Can you work these out from the model? Positions are in its coordinate system, mm. Face numbers are marked on the shaded views. A direction names the side the tool comes from. Give positions to 0.01 mm unless a question says otherwise; leave off trailing zeros. Write each loop counter-clockwise with the first axis right and the second up, starting at its lowest first coordinate (ties: lowest second). Pieces come first, ordered by that corner, then holes.
1. Suppose I cut it at D-D (y = -23.5). Please give me the cut outline in (x, z) (3 decimals).
2. Suppose I cut it at B-B (y = 0). Please give me the cut outline in (x, z) (3 decimals), and give its area (3 significant figures).
3. I'm going to push flat-ended pins straight in: pin 1 (11.5 mm diameter, centred on y = -14.5, z = -29, fed in from -X); pin 2 (18 mm diameter, centred on x = 13.5, y = -4, fed in from -Z) (3 decimals); pin 3 (20 mm diameter, centred on x = -42, y = -6.5, fed in from +Z); pin 4 (12 mm diameter, centred on x = -44, z = -33.5, fed in from -Y). Where does each tip first touch, or does it pass through?
4. Suppose I cut it at A-A (x = -23.5). Please give me the cut outline in (y, z) (3 decimals).
5. Suppose I cut it at C-C (x = 0). Please give me the cut outline in (y, z) (3 decimals).
6. On a 3-axis mill with a long thin cutter (end or side, diameter ignored), from which of +Z, -Z, +X, -X, +Y, -Y can I reach the whole of each face in a straight line? I mean the marked faces 1, 2 and 3. Say none if no direction works.
7. If I drill on probe 1 along Y at (x, z) = (-23.5, -1.95); probe 2 along X at (y, z) = (23.5, -1.85); probe 3 along X at (y, z) = (23.5, -1.6), over which ranges is the centre line in solid material (lowest first)?
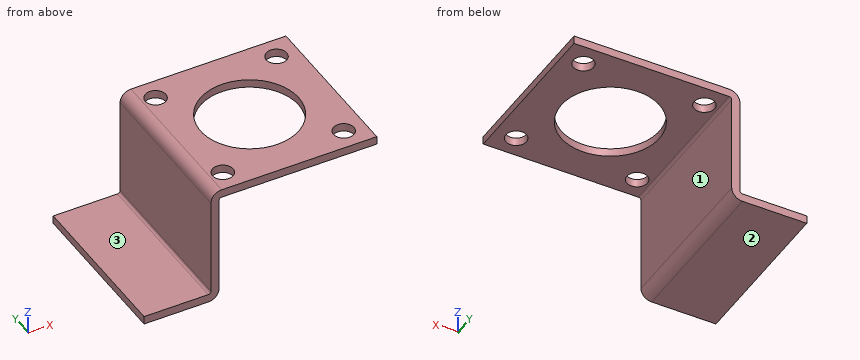
```python
from build123d import *

# Parameters (mm, degrees)
BOSS_EXTRUDE1_DEPTH     = 31.75
CUT_EXTRUDE1_DEPTH      = 82.262795763
CUT_EXTRUDE1_DEPTH_BACK = 82.262795763
SKETCH1_R               = 19.05
SKETCH1_R_2             = 4


with BuildPart() as part:
    # Sketch2 → Boss-Extrude1 (new, symmetric)
    with BuildSketch(Plane(origin=(0, 0, 0), x_dir=(1, 0, 0), z_dir=(0, 1, 0))):
        with BuildLine():
            Line((31.75, 0), (-28.499943, 0))
            ThreePointArc((-28.499943, 0), (-31.46342752, 1.22751548), (-32.690943, 4.191))
            Line((-32.690943, 4.191), (-32.690943, 42.208958))
            ThreePointArc((-32.690943, 42.208958), (-32.98852251, 42.92737849), (-33.706943, 43.224958))
            Line((-33.706943, 43.224958), (-58.673873, 43.224958))
            Line((-58.673873, 43.224958), (-58.673873, 46.399958))
            Line((-58.673873, 46.399958), (-33.706943, 46.399958))
            ThreePointArc((-33.706943, 46.399958), (-30.74345848, 45.17244252), (-29.515943, 42.208958))
            Line((-29.515943, 42.208958), (-29.515943, 4.191))
            ThreePointArc((-29.515943, 4.191), (-29.21836349, 3.47257951), (-28.499943, 3.175))
            Line((-28.499943, 3.175), (31.75, 3.175))
            Line((31.75, 3.175), (31.75, 0))
        make_face()
    extrude(amount=BOSS_EXTRUDE1_DEPTH, both=True)

    # Sketch1 → Cut-Extrude1 (cut, two sides: drawn at the far end of the back side and taken through both)
    with BuildSketch(Plane.XY.offset(-CUT_EXTRUDE1_DEPTH_BACK)):
        Circle(SKETCH1_R)
        with Locations((23.5, 23.5)):
            Circle(SKETCH1_R_2)
        with Locations((23.5, -23.5)):
            Circle(SKETCH1_R_2)
        with Locations((-23.5, -23.5)):
            Circle(SKETCH1_R_2)
        with Locations((-23.5, 23.5)):
            Circle(SKETCH1_R_2)
    extrude(amount=CUT_EXTRUDE1_DEPTH + CUT_EXTRUDE1_DEPTH_BACK, mode=Mode.SUBTRACT)


solid = part.part
```
Checks:
1. outline: (-58.674, -46.4) - (-33.707, -46.4) arc R4.191 ccw to (-29.516, -42.209) - (-29.516, -4.191) arc R1.016 cw to (-28.5, -3.175) - (-27.5, -3.175) - (-27.5, 0) - (-28.5, 0) arc R4.191 ccw to (-32.691, -4.191) - (-32.691, -42.209) arc R1.016 cw to (-33.707, -43.225) - (-58.674, -43.225) - close; (-19.5, -3.175) - (19.5, -3.175) - (19.5, 0) - (-19.5, 0) - close; (27.5, -3.175) - (31.75, -3.175) - (31.75, 0) - (27.5, 0) - close
2. outline: (-58.674, -46.4) - (-33.707, -46.4) arc R4.191 ccw to (-29.516, -42.209) - (-29.516, -4.191) arc R1.016 cw to (-28.5, -3.175) - (-19.05, -3.175) - (-19.05, 0) - (-28.5, 0) arc R4.191 ccw to (-32.691, -4.191) - (-32.691, -42.209) arc R1.016 cw to (-33.707, -43.225) - (-58.674, -43.225) - close; (19.05, -3.175) - (31.75, -3.175) - (31.75, 0) - (19.05, 0) - close
2. area: 296 mm2
3. pin 1: stops at x = -32.69
3. pin 2: stops at z = -3.175
3. pin 3: stops at z = -1.89
3. pin 4: passes through
4. outline: (-31.75, -3.175) - (-27.5, -3.175) - (-27.5, 0) - (-31.75, 0) - close; (-19.5, -3.175) - (19.5, -3.175) - (19.5, 0) - (-19.5, 0) - close; (27.5, -3.175) - (31.75, -3.175) - (31.75, 0) - (27.5, 0) - close
5. outline: (-31.75, -3.175) - (-19.05, -3.175) - (-19.05, 0) - (-31.75, 0) - close; (19.05, -3.175) - (31.75, -3.175) - (31.75, 0) - (19.05, 0) - close
6. face 1: -Z, +X, +Y, -Y
6. face 2: -Z, +X, -X, +Y, -Y
6. face 3: +Z, -X, +Y, -Y
7. probe 1: y = -31.75 to -27.5, -19.5 to 19.5, 27.5 to 31.75
7. probe 2: x = -31.98 to -27.5, -19.5 to 19.5, 27.5 to 31.75
7. probe 3: x = -31.79 to -27.5, -19.5 to 19.5, 27.5 to 31.75
